Build history of the part. All positions in model axes, mm. A direction names the side the tool comes from. Round coordinates to 2 decimals unless told otherwise and drop trailing zeros. Loops run counter-clockwise (first coordinate to the right, second up) from the corner with the lowest first, then second, coordinate; pieces in that order, holes last. Notation, with made-up numbers: (21.25, 24.5) -> (59.25, 24.5) arc R18 ccw to (59.25, 31.5) -> close; hole circle Ø7 at (-6, 86.5). An arc over 180 degrees is marked (long way). Put each result on its own line as item: value. Start each with the question number.
Item 1: Pull direction Z, two halves, no side cores. Call faces 4 (the cylindrical face through (-13.124, 4.696, 3.031)), 5 (the flat face through (-11, 5, -15.72)), 6 (the flat face through (-11, 5, 9.68)), 7 (the flat face through (1.501, 5, 0)): +Z half, -Z half, draft (parallel to the pull), parting line (faces both ways), or undercut.
Item 2: Tool access for faces 1 (the cylindrical face through (-3.556, 6.488, -12.501)), 2 (the flat face through (-4, 5, -8.481)), 3 (the flat face through (-14, 0, -9)): list every direction of +Z, -Z, +X, -X, +Y, -Y with a clear straight run to the whole face (end or side of a thin tool).
Item 3: Flat gauge pins, fed straight in: pin 1 Ø3 at (x, z) = (-20.72, -12.55) entering from -Y; pin 2 Ø3 at (x, z) = (-8, -8.5) entering from +Y (3 decimals). Where does each tip first touch, or does it go through?
Item 4: Cut at D-D, the plane x = -5.75. List the corners of the cut face in (y, z) (3 decimals), plus the area to 3 significant figures.
Item 5: Drill centre lines: probe 1 along Z at (x, y) = (0.25, 2.75); probe 2 along X at (y, z) = (2, 6.5); probe 3 along X at (y, z) = (4.5, -0.75). Where is each one in solid material? Low to high. Write a range as [from, to].
Item 6: Cut at A-A, the plane z = -6.5. List the corners of the cut face in (x, y) (1 decimal).
Item 7: Cut at C-C, the plane z = -0.75. List the corners of the cut face in (x, y) (1 decimal), plus the area to 3 significant figures.
Item 8: Cut at B-B, the plane y = 9. List the corners of the cut face in (x, z), plus the area to 3 significant figures.
```python
from build123d import *

# Parameters (mm, degrees)
BOSS_EXTRUDE1_DEPTH        = 9.525
F_8_32_TAPPED_HOLE1_D      = 3.4544
F_10_CLEARANCE_HOLE1_D     = 5.1054
F_10_CLEARANCE_HOLE1_DEPTH = 6.35


with BuildPart() as part:
    # Sketch1 → Boss-Extrude1 (new body)
    with BuildSketch(Plane(origin=(0, 0, 0), x_dir=(1, 0, 0), z_dir=(0, 1, 0))):
        with BuildLine():
            Line((1.500621967, 8.481252019), (1.500621967, -9.679747981))
            Line((1.500621967, -9.679747981), (-23.899378033, -9.679747981))
            Line((-23.899378033, -9.679747981), (-23.899378033, 15.720252019))
            Line((-23.899378033, 15.720252019), (1.500621967, 15.720252019))
            Line((1.500621967, 15.720252019), (1.500621967, 9.370252019))
            Line((1.500621967, 9.370252019), (-11.199378033, 9.370252019))
            ThreePointArc((-11.199378033, 9.370252019), (-12.879430115, -3.103466214), (-7.959010924, 8.481252019))
            Line((-7.959010924, 8.481252019), (1.500621967, 8.481252019))
        make_face()
    extrude(amount=BOSS_EXTRUDE1_DEPTH)

    # #8-32 Tapped Hole1 (through all)
    with Locations(Plane(origin=(0, 9.525, 0), x_dir=(1, 0, 0), z_dir=(0, 1, 0))):
        with Locations((-20.724378033, 12.545252019), (-1.674378033, -6.504747981)):
            Hole(F_8_32_TAPPED_HOLE1_D / 2)

    # Sketch4 → #10-24 Tapped Hole1 (revolve, cut)
    with BuildSketch(Plane(origin=(-1.674378033, 4.7625, -8.481252019), x_dir=(0, 1, 0), z_dir=(1, 0, 0))):
        Polygon((0, 0), (0, 12.316824014), (1.89865, 11.176), (1.89865, 0), align=None)
    revolve(axis=Axis((-1.674378033, 4.7625, -14.831252019), (0, 0, 1)), mode=Mode.SUBTRACT)

    # #10 Clearance Hole1
    with Locations(Plane(origin=(0, 0, -15.720252019), x_dir=(-1, 0, 0), z_dir=(0, 0, -1))):
        with Locations((1.674378033, 4.7625)):
            Hole(F_10_CLEARANCE_HOLE1_D / 2, depth=F_10_CLEARANCE_HOLE1_DEPTH)


solid = part.part
```
Reply:
1. face 4: undercut
1. face 5: -Z half
1. face 6: +Z half
1. face 7: draft
2. face 1: -Z
2. face 2: +X, +Y, -Y
2. face 3: +Z, -Z, +X, -X, -Y
3. pin 1: passes through
3. pin 2: stops at y = 9.525
4. outline: (0, -15.72) -> (9.525, -15.72) -> (9.525, -9.37) -> (0, -9.37) -> close; (0, -8.481) -> (9.525, -8.481) -> (9.525, -6.28) -> (0, -6.28) -> close; (0, 0.24) -> (9.525, 0.24) -> (9.525, 9.68) -> (0, 9.68) -> close
4. area: 171 mm^2
5. probe 1: z = [-15.72, -9.37], [-8.48, 9.68]
5. probe 2: x = [-23.9, -3.4], [0.05, 1.5]
5. probe 3: x = [-23.9, -17.13], [-5.27, -3.55], [0.21, 1.5]
6. outline: (-23.9, 0) -> (-16.5, 0) -> (-16.5, 9.5) -> (-23.9, 9.5) -> close; (-5.9, 0) -> (1.5, 0) -> (1.5, 9.5) -> (-5.9, 9.5) -> close; hole circle Ø3.8 at (-1.7, 4.8)
7. outline: (-23.9, 0) -> (-17.1, 0) -> (-17.1, 9.5) -> (-23.9, 9.5) -> close; (-5.3, 0) -> (1.5, 0) -> (1.5, 9.5) -> (-5.3, 9.5) -> close; hole circle Ø3.8 at (-1.7, 4.8)
7. area: 118 mm^2
8. outline: (-23.9, -15.72) -> (1.5, -15.72) -> (1.5, -9.37) -> (-11.2, -9.37) arc R6.35 cw (long way) to (-7.96, -8.48) -> (1.5, -8.48) -> (1.5, 9.68) -> (-23.9, 9.68) -> close; hole circle Ø3.45 at (-20.72, -12.55); hole circle Ø3.45 at (-1.67, 6.5)
8. area: 490 mm^2
